Source: CAD feature listing. Evaluate the final solid. Frame: model axes, mm. Round coordinates to 2 decimals unless told otherwise and drop trailing zeros. Order: outer loops, then holes, each group sorted by start corner. A loop starts at its lowest first (then second) coordinate and runs counter-clockwise, first axis right, second up. Notation, with made-up numbers: M -6.5,81 L 17.5,81 A23 ccw 17.5,111 Z; hole C -17,60 d3. An arc over 180 degrees is marked long. Use one line per item in the form item = value. Start each with the question number.
Q1. Section C-C (z = 51). Return the cut outline in (x, y), plus the area to 3 significant figures.
Q2. Contact query for flat-ended pins moving along their axis: pin 1 (1.5 mm diameter, centred on x = -2, z = 10, fed in from -Y); pin 2 (2 mm diameter, centred on x = -2, z = 44, fed in from +Y); pin 3 (1.5 mm diameter, centred on y = -2.5, z = 38.5, fed in from -X). Output: stop coordinate, or through.
Q3. Pull-direction query (Y, two-part tool) for faces 1 (the flat face through (2, -2, 65)), 2 (the cylindrical face through (1.438, -0.748, 32.049)), 3 (the cylindrical face through (-0.867, 3.905, 32.049)); classes: pulls with the +Y half, pulls with the -Y half, needs draft (parallel to the pull), parting line crosses it, or undercut.
Q4. Section A-A (x = 0). Return the cut outline in (y, z), plus the area to 3 significant figures.
Q5. Material intervals for probe 1 along Y at (x, z) = (0, 29); probe 2 along X at (y, z) = (1, 11.5); probe 3 along Y at (x, z) = (1.25, 16), sorted ascending.
Autodesk Inventor part; units mm, degrees
ref_plane "YZ Plane" through (0, 0, 0) normal (1, 0, 0) x (0, 1, 0)
ref_plane "XZ Plane" through (0, 0, 0) normal (0, 1, 0) x (-1, 0, 0)
ref_plane "XY Plane" through (0, 0, 0) normal (0, 0, 1) x (1, 0, 0)
sketch "スケッチ1" plane through (0, 0, 0) normal (0, 0, 1) x (1, 0, 0)
  circle A0 centre (0, 0) radius 4
  dimension "d0" = 8
extrude "押し出し1" add sketch "スケッチ1" along normal blind 65
sketch "スケッチ2" plane through (0, 0, 65) normal (0, 0, 1) x (1, 0, 0)
  point P0 (0, 0)
hole "穴1" at (0, 0, 65) direction (0, 0, -1) diameter 3.242 end through all
chamfer "面取り1" distance 0.3 angle 45 4 edges at (-4, 0, 65) (0, 1.621, 65) (0, 1.621, 0) (-4, 0, 0)
properties part number "p8l65ALshaft"
Results list:
q1.outline = C 0,0 d8; hole C 0,0 d3.24
q1.area = 42.0 mm2
q2.pin_1 = -3.8
q2.pin_2 = 3.87
q2.pin_3 = -3.6
q3.face_1 = needs draft
q3.face_2 = undercut
q3.face_3 = parting line crosses it
q4.outline = M -4,0.3 L -3.7,0 L -1.92,0 L -1.62,0.3 L -1.62,64.7 L -1.92,65 L -3.7,65 L -4,64.7 Z; M 1.62,0.3 L 1.92,0 L 3.7,0 L 4,0.3 L 4,64.7 L 3.7,65 L 1.92,65 L 1.62,64.7 Z
q4.area = 309 mm2
q5.probe_1 = -4 to -1.62, 1.62 to 4
q5.probe_2 = -3.87 to -1.28, 1.28 to 3.87
q5.probe_3 = -3.8 to -1.03, 1.03 to 3.8
